The listing builds one solid part. Answer for the finished solid, in the listing's coordinates (mm). Face numbers are marked on the shaded views. Round coordinates to 2 decimals unless told otherwise and drop trailing zeros. Write each loop counter-clockwise with the first axis right and the second up, starting at its lowest first coordinate (ties: lowest second). Pieces come first, ordered by that corner, then holes. Notation, with made-up numbers: (24.25, 81.5) - (37.25, 81.5) arc R12 ccw to (37.25, 99.5) - close; hole circle Ø10 at (-25.5, 11.25). An arc over 180 degrees is marked (long way). Use a Markdown table: item, result. Add a question column.
1) Determine the mould class of the marked faces 1 and 2 for opening direction X: +X half, -X half, draft (parallel to the pull), parting line (faces both ways), or undercut.
2) A cutting plane is placed at B-B (x = -251). Give the vertices of the cut face in (y, z), then the cut area to 3 significant figures.
3) Find the intervals of material crossed by probe 1 along X at (y, z) = (-4.5, -3); probe 2 along Z at (x, y) = (-308, -3.25); probe 3 along X at (y, z) = (-7.5, 0.5), in increasing order. Write a range as from..to.
4) A cutting plane is placed at C-C (y = -6.5). Give the vertices of the cut face in (x, z), then the cut area to 4 significant figures.
5) A cutting plane is placed at D-D (z = 37). Give the vertices of the cut face in (x, y).
6) A cutting plane is placed at A-A (z = -10). Give the vertices of the cut face in (x, y).
```python
from build123d import *

# Parameters (mm, degrees)
SKETCH6_W           = 150
SKETCH6_H           = 90
BOSS_EXTRUDE1_DEPTH = 10
SKETCH7_W           = 145
SKETCH7_H           = 85
CUT_EXTRUDE1_DEPTH  = 10
SKETCH2_W           = 45
SKETCH2_H           = 35
CUT_EXTRUDE2_DEPTH  = 10
SKETCH4_R           = 2.5
CUT_EXTRUDE3_DEPTH  = 10
SKETCH5_W           = 7
SKETCH5_H           = 1.5
CUT_EXTRUDE4_DEPTH  = 10
SKETCH3_W           = 12
SKETCH3_H           = 57
CUT_EXTRUDE5_DEPTH  = 10


with BuildPart() as part:
    # Sketch6 → Boss-Extrude1 (new body)
    with BuildSketch(Plane(origin=(0, 0, 0), x_dir=(1, 0, 0), z_dir=(0, 1, 0))):
        with Locations((-292.180819859, -3.647511649)):
            Rectangle(SKETCH6_W, SKETCH6_H)
    extrude(amount=-BOSS_EXTRUDE1_DEPTH)

    # Sketch7 → Cut-Extrude1 (cut)
    with BuildSketch(Plane(origin=(0, -5, 0), x_dir=(1, 0, 0), z_dir=(0, 1, 0))):
        with Locations((-292.180819859, -3.647511649)):
            Rectangle(SKETCH7_W, SKETCH7_H)
    extrude(amount=-CUT_EXTRUDE1_DEPTH, mode=Mode.SUBTRACT)

    # Sketch2 → Cut-Extrude2 (cut)
    with BuildSketch(Plane(origin=(0, 0, 0), x_dir=(1, 0, 0), z_dir=(0, 1, 0))):
        with Locations((-327.180819859, -13.647511649)):
            Rectangle(SKETCH2_W, SKETCH2_H)
    extrude(amount=-CUT_EXTRUDE2_DEPTH, mode=Mode.SUBTRACT)

    # Sketch4 → Cut-Extrude3 (cut)
    with BuildSketch(Plane(origin=(0, 0, 0), x_dir=(1, 0, 0), z_dir=(0, 1, 0))):
        with Locations(Location((-341.213762503, 29.627320544, 0), (0, 0, 270))):
            Circle(SKETCH4_R)
        with Locations(Location((-329.213762503, 29.627320544, 0), (0, 0, 270))):
            Circle(SKETCH4_R)
    extrude(amount=-CUT_EXTRUDE3_DEPTH, mode=Mode.SUBTRACT)

    # Sketch5 → Cut-Extrude4 (cut)
    with BuildSketch(Plane(origin=(0, 0, 0), x_dir=(1, 0, 0), z_dir=(0, 1, 0))):
        with Locations((-317.213762503, 29.627320544)):
            Rectangle(SKETCH5_W, SKETCH5_H)
    extrude(amount=-CUT_EXTRUDE4_DEPTH, mode=Mode.SUBTRACT)

    # Sketch3 → Cut-Extrude5 (cut)
    with BuildSketch(Plane(origin=(0, 0, 0), x_dir=(1, 0, 0), z_dir=(0, 1, 0))):
        with Locations((-250.680819859, -4.647511649)):
            Rectangle(SKETCH3_W, SKETCH3_H)
    extrude(amount=-CUT_EXTRUDE5_DEPTH, mode=Mode.SUBTRACT)


solid = part.part
```
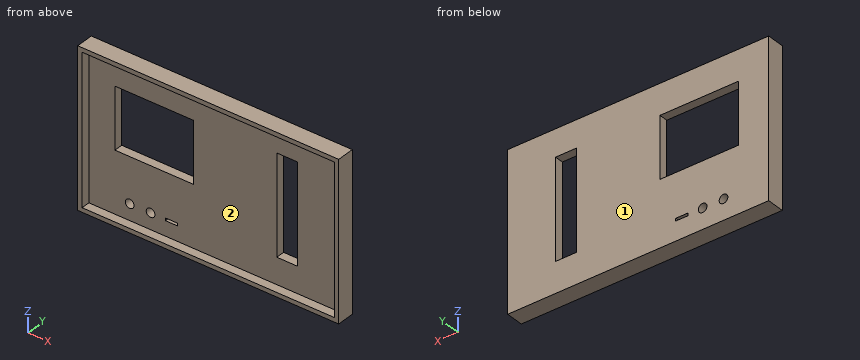
Entries:
| question | item | result |
|---|---|---|
| 1 | face 1 | draft |
| 1 | face 2 | undercut |
| 2 | outline | (-10, -41.35) - (0, -41.35) - (0, -23.85) - (-5, -23.85) - (-5, -38.85) - (-10, -38.85) - close; (-10, 46.15) - (-5, 46.15) - (-5, 33.15) - (0, 33.15) - (0, 48.65) - (-10, 48.65) - close |
| 2 | area | 190 mm² |
| 3 | probe 1 | x = -367.18..-349.68, -304.68..-256.68, -244.68..-217.18 |
| 3 | probe 2 | z = -41.35..-3.85, 31.15..48.65 |
| 3 | probe 3 | x = -367.18..-364.68, -219.68..-217.18 |
| 4 | outline | (-367.18, -41.35) - (-217.18, -41.35) - (-217.18, 48.65) - (-367.18, 48.65) - close; hole (-364.68, -38.85) - (-219.68, -38.85) - (-219.68, 46.15) - (-364.68, 46.15) - close |
| 4 | area | 1,175 mm² |
| 5 | outline | (-367.18, -10) - (-364.68, -10) - (-364.68, -5) - (-219.68, -5) - (-219.68, -10) - (-217.18, -10) - (-217.18, 0) - (-367.18, 0) - close |
| 6 | outline | (-367.18, -10) - (-364.68, -10) - (-364.68, -5) - (-256.68, -5) - (-256.68, 0) - (-367.18, 0) - close; (-244.68, -5) - (-219.68, -5) - (-219.68, -10) - (-217.18, -10) - (-217.18, 0) - (-244.68, 0) - close |
